Here's how the part is built. I have some questions about the finished solid (model axes, mm). Coordinates: 2 decimals unless noted, no trailing zeros. Write each loop counter-clockwise with the first axis right and the second up, starting at its lowest first coordinate (ties: lowest second). Pieces come first, ordered by that corner, then holes. Notation, with made-up numbers: (-12, 2.25) -> (-1, 2.25) arc R20 ccw to (-1, 15.25) -> close; hole circle Ø4 at (64, 3.25). An arc over 180 degrees is marked (long way). Use a Markdown table: item, result. Add a question column.
Item 1: Imagine slicing it at A-A, the plane z = -5.25. Write out the boundary of the cut face in (x, y), and give its area (3 significant figures).
Item 2: If I drill on line 1 along Z through (x, y) = (38, 13.25); line 2 along Z through (x, y) = (184.5, 10.5); line 3 along Z through (x, y) = (13, 7.5), over which ranges is the centre line in solid material (lowest first)? Write a range as from..to.
Item 3: Will these pins go through, and if not, where does the flat tip stop? pin 1 Ø4.5 at (x, y) = (11.81, 3.87) entering from -Z; pin 2 Ø6 at (x, y) = (101.81, 4.08) entering from +Z; pin 3 Ø1 at (x, z) = (144, -2) entering from +Y; pin 4 Ø2 at (x, z) = (152, -5.5) entering from +Y.
Item 4: Imagine slicing it at B-B, the plane x = 113. Write out the boundary of the cut face in (y, z), and give its area (3 significant figures).
```python
from build123d import *

# Parameters (mm, degrees)
BOSS_EXTRUDE1_DEPTH = 203.2
SKETCH2_R           = 2.38125
CUT_EXTRUDE1_DEPTH  = 205.198358087


with BuildPart() as part:
    # Sketch1 → Boss-Extrude1 (new body)
    with BuildSketch(Plane(origin=(0, 0, 0), x_dir=(0, 0, -1), z_dir=(1, 0, 0))):
        Polygon((0.083005599, 0.369350394), (0.083005599, 17.056692613), (1.083005599, 17.056692613), (1.083005599, 2.484301558), (8.052601156, 2.484301558), (8.052601156, 14.217769965), (3.483005599, 8.08145593), (3.483005599, 11.495503821), (7.624316401, 17.056692613), (10.84398523, 17.056692613), (10.84398523, 0.369350394), align=None)
    extrude(amount=BOSS_EXTRUDE1_DEPTH)

    # Sketch2 → Cut-Extrude1 (cut, through all)
    with BuildSketch(Plane.XY.offset(-0.083005599)):
        with Locations((11.814414866, 3.865442963)):
            Circle(SKETCH2_R)
        with Locations((191.596349419, 3.654678679)):
            Circle(SKETCH2_R)
        with Locations((101.810764284, 4.076207247)):
            Circle(SKETCH2_R)
    extrude(amount=-CUT_EXTRUDE1_DEPTH, mode=Mode.SUBTRACT)


solid = part.part
```
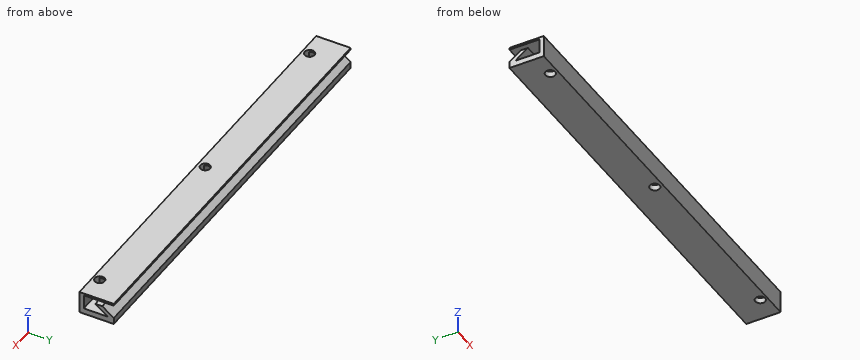
Ans:
| question | item | result |
|---|---|---|
| 1 | outline | (0, 0.37) -> (203.2, 0.37) -> (203.2, 2.48) -> (193.67, 2.48) arc R2.38 cw to (189.52, 2.48) -> (103.58, 2.48) arc R2.38 cw to (100.04, 2.48) -> (13.75, 2.48) arc R2.38 cw to (9.87, 2.48) -> (0, 2.48) -> close; (0, 10.45) -> (203.2, 10.45) -> (203.2, 13.87) -> (0, 13.87) -> close |
| 1 | area | 1,120 mm^2 |
| 2 | line 1 | z = -10.84..-8.05, -7.33..-4.79, -1.08..-0.08 |
| 2 | line 2 | z = -10.84..-8.05, -5.28..-3.48, -1.08..-0.08 |
| 2 | line 3 | z = -10.84..-8.05, -1.08..-0.08 |
| 3 | pin 1 | passes through |
| 3 | pin 2 | stops at z = -0.08 |
| 3 | pin 3 | stops at y = 2.48 |
| 3 | pin 4 | stops at y = 15.55 |
| 4 | outline | (0.37, -10.84) -> (17.06, -10.84) -> (17.06, -7.62) -> (11.5, -3.48) -> (8.08, -3.48) -> (14.22, -8.05) -> (2.48, -8.05) -> (2.48, -1.08) -> (17.06, -1.08) -> (17.06, -0.08) -> (0.37, -0.08) -> close |
| 4 | area | 93.5 mm^2 |
